from build123d import *

# Parameters (mm, degrees)
F0_W     = 500
F0_H     = 500
F1_DEPTH = 30
F2_SIZE  = 50
F4_DEPTH = 20


with BuildPart() as f1:
    # F0 (on Top) → F1 (new body)
    with BuildSketch(Plane.XY):
        Rectangle(F0_W, F0_H)
    extrude(amount=F1_DEPTH)

    # F2
    f2_edges = [f1.edges().sort_by_distance(p)[0] for p in [
        (250, -250, 15),
        (250, 250, 15),
        (-250, -250, 15),
        (-250, 250, 15),
    ]]
    chamfer(f2_edges, length=F2_SIZE)

    # F3 (on face) → F4 (cut)
    with BuildSketch(Plane(origin=(0, 0, 0), x_dir=(1, 0, 0), z_dir=(0, 0, -1))):
        with BuildLine():
            ThreePointArc((-35, -75), (0, -110), (35, -75))
            Line((35, -75), (35, 75))
            ThreePointArc((35, 75), (0, 110), (-35, 75))
            Line((-35, 75), (-35, -75))
        make_face()
    extrude(amount=-F4_DEPTH, mode=Mode.SUBTRACT)


solid = f1.part
The listing builds one solid part. Answer for the finished solid, in the listing's coordinates (mm). A direction names the side the tool comes from. Give positions to 0.01 mm unless a question says otherwise; leave off trailing zeros. Write each loop counter-clockwise with the first axis right and the second up, starting at its lowest first coordinate (ties: lowest second). Pieces come first, ordered by that corner, then holes.
1) Section C-C (y = -63.5) is taken. Write down the section's boundary in (x, z), and give its area (3 significant figures).
2) Find the intervals of material crossed by L1, parallel to X at y = 60, z = 6.5; L2, parallel to X at y = -204, z = 13; L3, parallel to Y at x = 217.5, z = 21, in increasing order.
3) For a pull along Y with two mould halves and no side action, classify faces 1 (the face through (-0.77, 109.99, 9.86)), 2 (the face through (225, -225, 15)), 3 (the face through (-3, 4, 30)) as pulls with the +Y half, pulls with the -Y half, needs draft (parallel to the pull), parting line crosses it, or undercut.
4) Section A-A (x = 0) is taken. Write down the section's boundary in (y, z), and give its area (3 significant figures).
5) Section B-B (z = 6) is taken. Write down the section's boundary in (x, y), and give its area (3 significant figures).
6) A tool of negligible diameter and unlimited length cuts with its end or side. For faces 4 (the face through (-250, -3, 15)), 5 (the face through (0.77, -109.99, 9.86)), from which of +Z, -Z, +X, -X, +Y, -Y can it reach the whole face along a straight path? Write none if from no direction.
Response:
1. outline: (-250, 0) - (-35, 0) - (-35, 20) - (35, 20) - (35, 0) - (250, 0) - (250, 30) - (-250, 30) - close
1. area: 13,600 mm2
2. L1: x = -250 to -35, 35 to 250
2. L2: x = -246 to 246
2. L3: y = -232.5 to 232.5
3. face 1: undercut
3. face 2: pulls with the -Y half
3. face 3: needs draft
4. outline: (-250, 0) - (-110, 0) - (-110, 20) - (110, 20) - (110, 0) - (250, 0) - (250, 30) - (-250, 30) - close
4. area: 10,600 mm2
5. outline: (-250, -200) - (-200, -250) - (200, -250) - (250, -200) - (250, 200) - (200, 250) - (-200, 250) - (-250, 200) - close; hole (-35, -75) arc R35 ccw to (35, -75) - (35, 75) arc R35 ccw to (-35, 75) - close
5. area: 231,000 mm2
6. face 4: +Z, -Z, -X, +Y, -Y
6. face 5: -Z
